Read the model definition and answer for the solid it produces. Units are mm, in the model's axes. A direction names the side the tool comes from. Coordinates: 2 decimals unless noted, no trailing zeros. Loops run counter-clockwise (first coordinate to the right, second up) from the corner with the lowest first, then second, coordinate; pieces in that order, holes last. Notation, with made-up numbers: (53.25, 9) -> (104.25, 9) arc R10 cw to (104.25, 26) -> close; hole circle Ø8 at (71, -30). An arc over 180 degrees is marked (long way). Answer in a Markdown table with one row per item.
Autodesk Inventor part; units mm, degrees
ref_plane "YZ Plane" through (0, 0, 0) normal (1, 0, 0) x (0, 1, 0)
ref_plane "XZ Plane" through (0, 0, 0) normal (0, 1, 0) x (-1, 0, 0)
ref_plane "XY Plane" through (0, 0, 0) normal (0, 0, 1) x (1, 0, 0)
sketch "Sketch1" plane through (0, 0, 0) normal (0, 1, 0) x (-1, 0, 0)
  circle A0 centre (0, 0) radius 12
  dimension "d0" = 24
extrude "Extrusion1" add sketch "Sketch1" along normal blind 24
sketch "Sketch2" plane through (0, 24, 0) normal (0, 1, 0) x (1, 0, 0)
  circle A0 centre (0, 0) radius 9
  dimension "d3" = 18
extrude "Extrusion2" add sketch "Sketch2" along normal blind 4
sketch "Sketch3" plane through (0, 28, 0) normal (0, 1, 0) x (1, 0, 0)
  circle A0 centre (0, 0) radius 1
  circle A1 centre (0, 0) radius 1.5
  dimension "d6" = 2
  dimension "d7" = 3
extrude "Extrusion3" add sketch "Sketch3" along normal blind 2
sketch "Sketch4" plane through (0, 28, 0) normal (0, 1, 0) x (1, 0, 0)
  circle A0 centre (0, 0) radius 1
extrude "Extrusion4" add sketch "Sketch4" along normal blind 8
sketch "Sketch5" plane through (0, 0, 0) normal (0, -1, 0) x (1, 0, 0)
  circle A0 centre (0, 0) radius 9
  circle A1 centre (0, 9) radius 1
  circle A2 centre (0, -9) radius 1
  line L0 (0.9985, 8.9444) -> (-0.9985, 8.9444)
  line L1 (0.9985, 9.0556) -> (-0.9985, 9.0556)
  line L2 (0.9985, -8.9444) -> (-0.9985, -8.9444)
  line L3 (0.9985, -9.0556) -> (-0.9985, -9.0556)
  dimension "d12" = 2
  dimension "d13" = 2
extrude "Extrusion5" add sketch "Sketch5" along normal blind 3 contours L0 A0 | A0 A1 L1 | A2 L3 A0 | A0 L2
sketch "Sketch6" plane through (0, 0, 0) normal (0, -1, 0) x (1, 0, 0)
  circle A0 centre (0, 0) radius 1.5
  circle A1 centre (0, 0) radius 2
  dimension "d16" = 4
extrude "Extrusion6" add sketch "Sketch6" along normal blind 1 contours A0 | A1
sketch "Sketch7" plane through (0, -1, 0) normal (0, -1, 0) x (1, 0, 0)
  circle A0 centre (0, 0) radius 1
  dimension "d19" = 2
extrude "Extrusion7" add sketch "Sketch7" along normal blind 0.2
sketch "Sketch8" plane through (0, 28, 0) normal (0, 1, 0) x (1, 0, 0)
  circle A0 centre (0, 5) radius 1
  circle A1 centre (0, -5) radius 1
  point P0 (0, 0)
  dimension "d22" = 2
  dimension "d23" = 2
extrude "Extrusion8" cut sketch "Sketch8" against normal blind 2
sketch "Sketch9" plane through (0.9985, 0, -9.0556) normal (0, 0, -1) x (-1, 0, 0)
  point P0 (0.9985, 0)
equation "\"BendRadius\" = Thickness"
equation "\"BendReliefWidth\" = Thickness"
equation "\"BendReliefDepth\" = 0.5 * Thickness"
equation "\"CornerReliefSize\" = 4 * Thickness"
equation "\"MinimumRemnant\" = 2 * Thickness"
equation "\"TransitionRadius\" = BendRadius"
equation "\"JacobiRadiusSize\" = BendRadius"
equation "\"GapSize\" = Thickness"
1. A cutting plane is placed at D-D on z = 3.5. Give the vertices of the cut face in (x, y), and give its area (3 significant figures).
A:
| item | result |
|---|---|
| outline | (-11.48, 0) -> (11.48, 0) -> (11.48, 24) -> (8.29, 24) -> (8.29, 28) -> (-8.29, 28) -> (-8.29, 24) -> (-11.48, 24) -> close |
| area | 617 mm2 |
2. The mould has two halves that part along X. Classify faces 4 (the cylindrical face through (11.99, 11.83, -0.53)), 5 (the flat face through (0, -1.2, 0)), 6 (the flat face through (0, 26, 5)), 7 (the flat face through (0, 26, -5)): pulls with the +X half, pulls with the -X half, needs draft (parallel to the pull), parting line crosses it, or undercut.
A:
| item | result |
|---|---|
| face 4 | parting line crosses it |
| face 5 | needs draft |
| face 6 | undercut |
| face 7 | undercut |
3. Given pin 1 Ø5 at (y, z) = (19, 4.5) entering from -X; pin 2 Ø6 at (x, y) = (-3, 30.5) entering from -Z; pin 3 Ø12 at (x, z) = (8.5, 0.5) entering from +Y, each flat-ended and moving along its own axis, determine where each tip first touches the part or whether it passes through.
A:
| item | result |
|---|---|
| pin 1 | stops at x = -11.83 |
| pin 2 | stops at z = -8.9 |
| pin 3 | stops at y = 28 |
4. A cutting plane is placed at A-A on z = 0. Give the vertices of the cut face in (x, y), and give its area (3 significant figures).
A:
| item | result |
|---|---|
| outline | (-12, 0) -> (-2, 0) -> (-2, -1) -> (-1, -1) -> (-1, -1.2) -> (1, -1.2) -> (1, -1) -> (2, -1) -> (2, 0) -> (12, 0) -> (12, 24) -> (9, 24) -> (9, 28) -> (1.5, 28) -> (1.5, 30) -> (1, 30) -> (1, 36) -> (-1, 36) -> (-1, 30) -> (-1.5, 30) -> (-1.5, 28) -> (-9, 28) -> (-9, 24) -> (-12, 24) -> close |
| area | 670 mm2 |
5. A tool of negligible diameter and unlimited length cuts with its end or side. For faces 1 (the flat face through (1, -1, -1)), 2 (the flat face through (-2, 24, 9)), 3 (the flat face through (0, 36, 0)), from which of +Z, -Z, +X, -X, +Y, -Y can it reach the whole face along a straight path? Write none if from no direction.
A:
| item | result |
|---|---|
| face 1 | -Y |
| face 2 | +Y |
| face 3 | +Z, -Z, +X, -X, +Y |
6. Find the intervals of material crossed by probe 1 along Z at (x, y) = (0, 27.45); probe 2 along Y at (x, z) = (-7.5, 2); probe 3 along X at (y, z) = (27.2, 5), in increasing order.
A:
| item | result |
|---|---|
| probe 1 | z = -9 to -6, -4 to 4, 6 to 9 |
| probe 2 | y = 0 to 28 |
| probe 3 | x = -7.48 to -1, 1 to 7.48 |
7. A cutting plane is placed at C-C on y = 20.5. Give the vertices of the cut face in (x, z).
A:
| item | result |
|---|---|
| outline | circle Ø24 at (0, 0) |
8. A cutting plane is placed at B-B on x = 3.25. Give the vertices of the cut face in (y, z), and give its area (3 significant figures).
A:
| item | result |
|---|---|
| outline | (0, -11.55) -> (24, -11.55) -> (24, -8.39) -> (28, -8.39) -> (28, 8.39) -> (24, 8.39) -> (24, 11.55) -> (0, 11.55) -> close |
| area | 622 mm2 |
